from build123d import *

# Parameters (mm, degrees)
SKETCH1_W           = 57.15
SKETCH1_H           = 31.75
BOSS_EXTRUDE1_DEPTH = 28.575
SKETCH2_R           = 12.573
CUT_EXTRUDE1_DEPTH  = 72.349251047
SKETCH3_W           = 2.54
SKETCH3_H           = 28.575
BOSS_EXTRUDE2_DEPTH = 31.75
SKETCH4_R           = 9.525
CUT_EXTRUDE2_DEPTH  = 2.54
BOSS_EXTRUDE3_DEPTH = 28.575
SKETCH6_R           = 2.032
CUT_EXTRUDE3_DEPTH  = 12.7


with BuildPart() as part:
    # Sketch1 → Boss-Extrude1 (new body)
    with BuildSketch(Plane.XY):
        with Locations((28.575, 15.875)):
            Rectangle(SKETCH1_W, SKETCH1_H)
    extrude(amount=-BOSS_EXTRUDE1_DEPTH)

    # Sketch2 → Cut-Extrude1 (cut, through all)
    with BuildSketch(Plane.ZY):
        with Locations((-15.875, 15.875)):
            Circle(SKETCH2_R)
    extrude(amount=-CUT_EXTRUDE1_DEPTH, mode=Mode.SUBTRACT)

    # Sketch3 → Boss-Extrude2 (add)
    with BuildSketch(Plane(origin=(0, 31.75, 0), x_dir=(1, 0, 0), z_dir=(0, 1, 0))):
        with Locations((-1.27, 14.2875)):
            Rectangle(SKETCH3_W, SKETCH3_H)
    extrude(amount=-BOSS_EXTRUDE2_DEPTH)

    # Sketch4 → Cut-Extrude2 (cut)
    with BuildSketch(Plane.ZY.offset(2.54)):
        with Locations((-15.875, 15.875)):
            Circle(SKETCH4_R)
    extrude(amount=-CUT_EXTRUDE2_DEPTH, mode=Mode.SUBTRACT)

    # Sketch5 → Boss-Extrude3 (add)
    with BuildSketch(Plane.XY):
        Polygon((-2.54, 0), (57.15, 0), (57.15, -15.993887296), align=None)
    extrude(amount=-BOSS_EXTRUDE3_DEPTH)

    # Sketch6 → Cut-Extrude3 (cut)
    with BuildSketch(Plane(origin=(57.15, 0, 0), x_dir=(0, 0, -1), z_dir=(1, 0, 0))):
        with Locations((3.175, 28.575)):
            Circle(SKETCH6_R)
        with Locations((25.4, 28.575)):
            Circle(SKETCH6_R)
        with Locations((25.4, -3.293887296)):
            Circle(SKETCH6_R)
        with Locations((3.175, -3.293887296)):
            Circle(SKETCH6_R)
    extrude(amount=-CUT_EXTRUDE3_DEPTH, mode=Mode.SUBTRACT)


solid = part.part
Geometry check sheet. Reference: the model listing, model coordinates, mm. A direction names the side the tool comes from. Give positions to 0.01 mm unless a question says otherwise; leave off trailing zeros. Order: outer loops, then holes, each group sorted by start corner. A loop starts at its lowest first (then second) coordinate and runs counter-clockwise, first axis right, second up.
1) Material ranges on probe 1 along Z at (x, y) = (49.5, -3.5) (3 decimals); probe 2 along Y at (x, z) = (42, -17.75); probe 3 along Z at (x, y) = (32.5, 26) (3 decimals), recorded low to high.
Results are:
probe 1: z = -28.575 to -27.422, -23.378 to -5.197, -1.153 to 0
probe 2: y = -11.93 to 3.44, 28.31 to 31.75
probe 3: z = -28.575 to -23.329, -8.421 to 0
2) Cross-section at B-B (y = 8). Record the boundary of the cut face in (x, z) (3 decimals), then the cut area to 3 significant figures.
Results are:
outline: (-2.54, -28.575) - (57.15, -28.575) - (57.15, -25.676) - (0, -25.676) - (0, -21.233) - (-2.54, -21.233) - close; (-2.54, -10.517) - (0, -10.517) - (0, -6.074) - (57.15, -6.074) - (57.15, 0) - (-2.54, 0) - close
area: 558 mm2
3) Cross-section at C-C (x = 51). Record the boundary of the cut face in (y, z) (3 decimals).
Results are:
outline: (-14.346, -28.575) - (31.75, -28.575) - (31.75, 0) - (-14.346, 0) - close; hole circle Ø4.064 at (-3.294, -25.4); hole circle Ø4.064 at (-3.294, -3.175); hole circle Ø25.146 at (15.875, -15.875); hole circle Ø4.064 at (28.575, -25.4); hole circle Ø4.064 at (28.575, -3.175)
4) Cross-section at D-D (z = -2). Record the boundary of the cut face in (x, y).
Results are:
outline: (-2.54, 0) - (57.15, -15.99) - (57.15, -4.95) - (44.45, -4.95) - (44.45, -1.64) - (57.15, -1.64) - (57.15, 26.92) - (44.45, 26.92) - (44.45, 30.23) - (57.15, 30.23) - (57.15, 31.75) - (-2.54, 31.75) - close
5) Tool access check on faces 5 (the cylindrical face through (50.889, -4.072, -5.052)), 6 (the flat face through (57.15, 3, -14)). Record the directions out of +Z, -Z, +X, -X, +Y, -Y that give a thin tool (end or side, any length) a straight path to the whole face; none if there is none.
Results are:
face 5: +X
face 6: +Z, -Z, +X, +Y, -Y
6) Cross-section at A-A (z = -15.5). Record the boundary of the cut face in (x, y).
Results are:
outline: (-2.54, 0) - (57.15, -15.99) - (57.15, 3.31) - (0, 3.31) - (0, 6.36) - (-2.54, 6.36) - close; (-2.54, 25.39) - (0, 25.39) - (0, 28.44) - (57.15, 28.44) - (57.15, 31.75) - (-2.54, 31.75) - close
7) Gauge pin test, flat ends, axial feed: pin 1 (12 mm diameter, centred on y = 13.5, z = -20, fed in from +X); pin 2 (2 mm diameter, centred on x = 31, z = -15, fed in from -Y); pin 3 (1.2 mm diameter, centred on y = -4, z = -25, fed in from +X). Record the tip position at first contact, or that the pin passes through.
Results are:
pin 1: stops at x = 0
pin 2: stops at y = -9.25
pin 3: stops at x = 44.45
8) Draft check along Y on faces 1 (the cylindrical face through (50.889, 29.185, -27.338)), 2 (the flat face through (28, 14, -28.575)), 3 (the flat face through (27.72, -8.11, -14.09)), 4 (the flat face through (44.45, 29, -3)). Enter one of: released by +Y, released by -Y, zero draft, split by the parting line, or undercut.
Results are:
face 1: undercut
face 2: zero draft
face 3: released by -Y
face 4: undercut
